Here's how the part is built. I have some questions about the finished solid (model axes, mm). Face numbers are marked on the shaded views. A direction names the side the tool comes from. Give positions to 0.01 mm unless a question says otherwise; leave off trailing zeros. Order: outer loops, then holes, each group sorted by start corner. A loop starts at its lowest first (then second) coordinate and runs counter-clockwise, first axis right, second up. Notation, with made-up numbers: M 18.25,35 L 39.25,35 A13 cw 39.25,48 Z; hole C 88.5,87 d9. An arc over 180 degrees is marked long. Use one line per item in the form item = value.
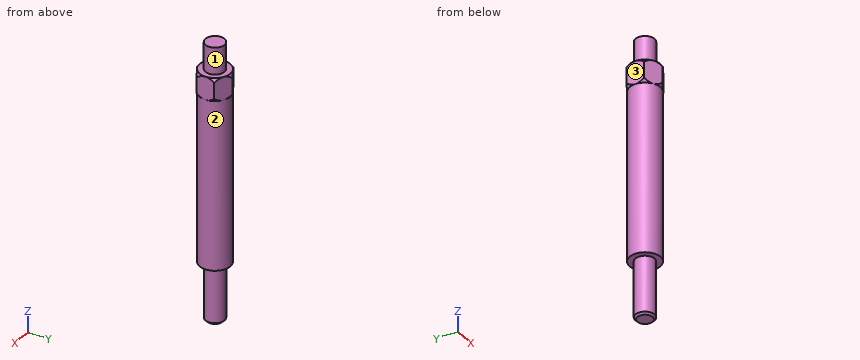
Autodesk Inventor part; units mm, degrees
ref_plane "YZ Plane" through (0, 0, 0) normal (1, 0, 0) x (0, 1, 0)
ref_plane "XZ Plane" through (0, 0, 0) normal (0, 1, 0) x (-1, 0, 0)
ref_plane "XY Plane" through (0, 0, 0) normal (0, 0, 1) x (1, 0, 0)
sketch "Sketch1" plane through (0, 0, 0) normal (0, 0, 1) x (1, 0, 0)
  circle A0 centre (0, 0) radius 4
  line L0 (-4, 2.3094) -> (0, 4.6188)
  line L1 (0, 4.6188) -> (4, 2.3094)
  line L2 (4, 2.3094) -> (4, -2.3094)
  line L3 (4, -2.3094) -> (0, -4.6188)
  line L4 (0, -4.6188) -> (-4, -2.3094)
  line L5 (-4, -2.3094) -> (-4, 2.3094)
  point P0 (-4, 0)
  dimension "d0" = 8
extrude "Extrusion1" add sketch "Sketch1" along normal blind 6
sketch "Sketch2" plane through (0, 0, 6) normal (0, 0, 1) x (1, 0, 0)
  circle A0 centre (0, 0) radius 4
extrude "Extrusion2" cut sketch "Sketch2" against normal blind 6 draft 35 keep common part
extrude "Extrusion3" cut sketch "Sketch1" along normal blind 6 draft 35 contours A0 keep common part
sketch "Sketch3" plane through (0, 0, 0) normal (1, 0, 0) x (0, 1, 0)
  line L0 (0, 0) -> (-3.4641, 0)
  line L1 (0, 0) -> (0, -59)
  line L2 (0, -59) -> (2, -59)
  line L3 (2.5, -58.5) -> (2.5, -44)
  line L4 (2.5, -44) -> (4, -44)
  line L5 (4, -44) -> (4, 0)
  line L6 (0, 0) -> (27.6878, 0) construction
  line L7 (3.4641, 0) -> (0, 0)
  line L8 (4, 0) -> (0, 0)
  line L9 (2.5, -58.5) -> (2, -59)
  point P0 (2.5, -59)
  dimension "d7" = 4
  dimension "d8" = 2.5
  dimension "d9" = 44
  dimension "d10" = 15
  dimension "d11" = 0.5
  dimension "d12" = 0.5
revolve "Revolution1" add sketch "Sketch3" angle 360 about axis through (0, 0, 0) along (0, 0, -1)
sketch "Sketch4" plane through (0, 0, 6) normal (0, 0, 1) x (1, 0, 0)
  circle A0 centre (0, 0) radius 2
  circle A1 centre (0, 0) radius 2.5
  point P0 (0, 0)
  dimension "d14" = 5
extrude "Extrusion4" add sketch "Sketch4" along normal blind 7 contours A0 | A1
thread "Thread1"
thread "Thread2"
properties part number "Component 9 (Suspension Spacer)"
Q1. I need wall thicknesses on L1, parallel to X at y = 1.5, z = -55; L2, parallel to X at y = -0.25, z = -27.5; L3, parallel to Z at x = 0.75, y = 3.25. Which ranges of each line are inside material? Lowest first, please.
Found:
L1 = -2 to 2
L2 = -3.99 to 3.99
L3 = -44 to 6
Q2. I'm going to push flat-ended pins straight in: pin 1 Ø1 at (x, z) = (0.5, -18) entering from -Y; pin 2 Ø1.5 at (x, z) = (2.5, -47) entering from -Y; pin 3 Ø1 at (y, z) = (3.5, -43) entering from +X. Where does each tip first touch, or does it pass through?
Found:
pin_1 = -4
pin_2 = -1.79
pin_3 = 2.65
Q3. On a 3-axis mill with a long thin cutter (end or side, diameter ignored), from which of +Z, -Z, +X, -X, +Y, -Y can I reach the whole of each face in a straight line? I mean the marked faces 1, 2 and 3. Say none if no direction works.
Found:
face_1 = +Z
face_2 = -Z
face_3 = +Z, -Z, -X, +Y, -Y
Q4. I want a section at A-A on z = -10. Write out the boundary of the cut face in (x, y).
Found:
outline = C 0,0 d8
